```python
from build123d import *

# Parameters (mm, degrees)
F1_DEPTH      = 19.05
F2_W          = 26.162
F2_H          = 57.15
F3_DEPTH      = 38.101
F3_DEPTH_BACK = 38.101
F4_R          = 9.525
F5_DEPTH      = 19.051
F6_R          = 9.525
F6_R_2        = 8.255
F7_DEPTH      = 1.778


with BuildPart() as f1:
    # F0 (on Front) → F1 (new body)
    with BuildSketch(Plane.XZ):
        with BuildLine():
            Line((-38.1, -43.3179386414), (-38.1, -49.6679386414))
            Line((-38.1, -49.6679386414), (38.1, -49.6679386414))
            Line((38.1, -49.6679386414), (38.1, -43.3179386414))
            Line((38.1, -43.3179386414), (22.225, -43.3179386414))
            ThreePointArc((22.225, -43.3179386414), (17.7348719395, -41.458066702), (15.875, -36.9679386414))
            Line((15.875, -36.9679386414), (15.875, 7.4820613586))
            ThreePointArc((15.875, 7.4820613586), (14.0151280605, 11.9721894191), (9.525, 13.8320613586))
            Line((9.525, 13.8320613586), (-9.525, 13.8320613586))
            ThreePointArc((-9.525, 13.8320613586), (-14.0151280605, 11.9721894191), (-15.875, 7.4820613586))
            Line((-15.875, 7.4820613586), (-15.875, -36.9679386414))
            ThreePointArc((-15.875, -36.9679386414), (-17.7348719395, -41.458066702), (-22.225, -43.3179386414))
            Line((-22.225, -43.3179386414), (-38.1, -43.3179386414))
        make_face()
    extrude(amount=F1_DEPTH)

    # F2 (on Right) → F3 (cut, two sides)
    with BuildSketch(Plane.YZ) as f3_sk:
        with Locations((-0.254, -14.7429386414)):
            Rectangle(F2_W, F2_H)
    extrude(amount=-F3_DEPTH, mode=Mode.SUBTRACT)
    extrude(f3_sk.sketch, amount=F3_DEPTH_BACK, mode=Mode.SUBTRACT)

    # F4 (on face) → F5 (cut, through all)
    with BuildSketch(Plane.XZ.offset(19.05)):
        with Locations((0, -2.0429386414)):
            Circle(F4_R)
    extrude(amount=-F5_DEPTH, mode=Mode.SUBTRACT)

    # F6 (on face) → F7 (join)
    with BuildSketch(Plane(origin=(0, -13.335, 0), x_dir=(-1, 0, 0), z_dir=(0, 1, 0))):
        with Locations((0, -2.0429386414)):
            Circle(F6_R)
        with Locations((0, -2.0429386414)):
            Circle(F6_R_2, mode=Mode.SUBTRACT)
    extrude(amount=-F7_DEPTH)


solid = f1.part
```
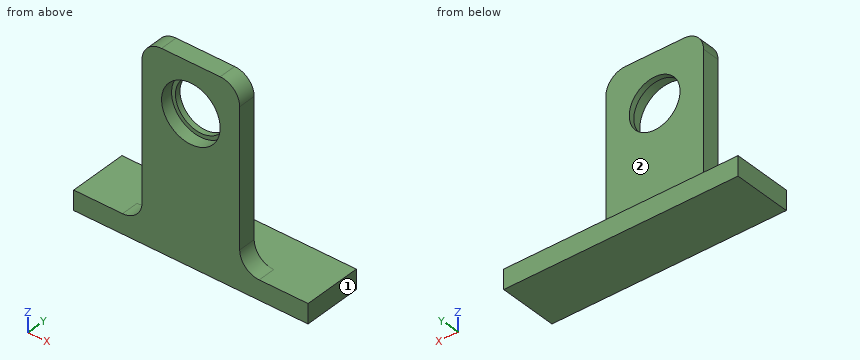
CAD build for the part. Positions are in the model's coordinates, mm. Face numbers are marked on the shaded views. A direction names the side the tool comes from. Round coordinates to 2 decimals unless told otherwise and drop trailing zeros. Loops run counter-clockwise (first coordinate to the right, second up) from the corner with the lowest first, then second, coordinate; pieces in that order, holes last. Notation, with made-up numbers: M 43,31 L 52,31 A22 ccw 52,59 Z; hole C 14,-29 d2. An arc over 180 degrees is marked long. Return JSON: item names as keys, results as strings. Group by question number.
(1) Tool access for the marked faces 1 and 2: list every direction of +Z, -Z, +X, -X, +Y, -Y with a clear straight run to the whole face (end or side of a thin tool).
(2) Saw through at B-B, the plane z = -6.5. List the corners of the cut face in (x, y) (3 decimals).
(3) Saw through at A-A, the plane x = 0. List the corners of the cut face in (y, z) (3 decimals), and give its area (3 significant figures).
(4) Wall check: probe 1 along Z at (x, y) = (0, -13.85); probe 2 along Z at (x, y) = (0, -16.15); probe 3 along Y at (x, z) = (-14, -1) (3 decimals). Give the ranges that are in metal, low to high. Write a range as [from, to].
(5) Drop flat-ended pins along their axis: P1, Ø5, axis at y = -8.5, z = -5.5, coming from the -X side; P2, Ø25, axis at x = 0, z = -2.04, coming from the +Y side (3 decimals); P3, Ø5, axis at y = -5, z = -41, coming from the -X side; P4, Ø6.5, axis at y = -17.5, z = -4.5, coming from the -X side (3 decimals). Give the stop position or say it passes through.
(6) Saw through at D-D, the plane x = 33.5. List the corners of the cut face in (y, z).
(7) Saw through at C-C, the plane y = -1.25. List the corners of the cut face in (x, z).
Answer list:
{
 "1": {"face 1": "+Z, -Z, +X, +Y, -Y", "face 2": "+Z, +X, -X, +Y"},
 "2": {"outline": "M -15.875,-19.05 L -8.418,-19.05 L -8.418,-15.113 L -6.948,-15.113 L -6.948,-13.335 L -15.875,-13.335 Z; M 6.948,-15.113 L 8.418,-15.113 L 8.418,-19.05 L 15.875,-19.05 L 15.875,-13.335 L 6.948,-13.335 Z"},
 "3": {"outline": "M -19.05,-49.668 L 0,-49.668 L 0,-43.318 L -13.335,-43.318 L -13.335,-10.298 L -15.113,-10.298 L -15.113,-11.568 L -19.05,-11.568 Z; M -19.05,7.482 L -15.113,7.482 L -15.113,6.212 L -13.335,6.212 L -13.335,13.832 L -19.05,13.832 Z", "area": "343 mm2"},
 "4": {"probe 1": "[-49.67, -10.3], [6.21, 13.83]", "probe 2": "[-49.67, -11.57], [7.48, 13.83]", "probe 3": "[-19.05, -13.335]"},
 "5": {"P1": "through", "P2": "y = -13.335", "P3": "x = -38.1", "P4": "x = -15.875"},
 "6": {"outline": "M -19.05,-49.67 L 0,-49.67 L 0,-43.32 L -19.05,-43.32 Z"},
 "7": {"outline": "M -38.1,-49.67 L 38.1,-49.67 L 38.1,-43.32 L -38.1,-43.32 Z"}
}
